from build123d import *

# Parameters (mm, degrees)
F1_DEPTH    = 200
F2_R        = 15
F4_DEPTH    = 15
F5_W        = 259.7017054144
F5_H        = 160
F6_DEPTH    = 50
F7_T1_DEPTH = 160
F8_R        = 15
F9_DEPTH    = 300


# Not quite as in the source:
# - a fillet or chamfer that OpenCascade refuses, or shapes differently, is made with other operations: its cross-section is extruded or revolved along the edge and cut away or added


with BuildPart() as f1:
    # F0 (on Front) → F1 (new body)
    with BuildSketch(Plane.XZ):
        with BuildLine():
            add(Edge.make_bspline(
                [(20.2008041868, 100), (146.0822657859, 99.5052919304), (265.431836351, 89.8162356005), (400, 75.4941478372)],
                knots=[0.5253173238, 0.5253173238, 0.5253173238, 0.5253173238, 1, 1, 1, 1], degree=3))
            Line((20.2008041868, 100), (0, 100))
            add(Edge.make_bspline(
                [(-400, 75.4941478372), (-275.3232982272, 88.4775108691), (-133.3944766528, 99.4743507493), (0, 100)],
                knots=[0, 0, 0, 0, 0.5, 0.5, 0.5, 0.5], degree=3))
            Line((-400, 75.4941478372), (-400, 44.4300249219))
            add(Edge.make_bspline(
                [(-41.6261814535, 0), (-214.6242707968, 0), (-393.6260249555, 49.33328574), (-400, 44.4300249219)],
                knots=[0, 0, 0, 0, 0.9473133281, 0.9473133281, 0.9473133281, 0.9473133281], degree=3))
            Line((-41.6261814535, 0), (209.8438292742, -64.8676306009))
            Line((209.8438292742, -64.8676306009), (266.6716873646, 0))
            add(Edge.make_bspline(
                [(400, 75.4941478372), (313.5865926743, 36.6108752787), (291.246175766, 29.9087464809), (266.6716873646, 0)],
                knots=[0, 0, 0, 0, 153.2181624608, 153.2181624608, 153.2181624608, 153.2181624608], degree=3))
        make_face()
    extrude(amount=F1_DEPTH)

    # F2
    f2_edges = [f1.edges().sort_by_distance(p)[0] for p in [
        (-200.289149, -200, 92.61289),
        (210.407204, -200, 92.68637),
        (-200.289149, 0, 92.61289),
        (10.100402, -200, 100),
        (10.100402, 0, 100),
        (210.407204, 0, 92.68637),
    ]]
    fillet(f2_edges, radius=F2_R)

    # F3 (on face) → F4 (cut, symmetric)
    with BuildSketch(Plane(origin=(150.8768626718, 0, -132.1770020211), x_dir=(0, 1, 0), z_dir=(0.7521818814, 0, -0.6589555503))):
        with BuildLine():
            Line((-180, 226.1682897806), (-180, 89.4854995586))
            Line((-180, 89.4854995586), (-20, 89.4854995586))
            Line((-20, 89.4854995586), (-20, 226.1682897806))
            add(Edge.make_bspline(
                [(-180, 226.1682897806), (-153.3333333333, 247.7404251695), (-100, 290.8846959472), (-46.6666666667, 247.7404251695), (-20, 226.1682897806)],
                knots=[0, 0, 0, 0, 0.5, 1, 1, 1, 1], degree=3))
        make_face()
    extrude(amount=F4_DEPTH, both=True, mode=Mode.SUBTRACT)

    # F5 (on face) → F6 (cut)
    with BuildSketch(Plane(origin=(-2.5970065182, 0, -10.0677217734), x_dir=(0.9683032706, 0, -0.2497774533), z_dir=(-0.2497774533, 0, -0.9683032706))):
        with Locations((89.5440850641, 100)):
            Rectangle(F5_W, F5_H)
    extrude(amount=-F6_DEPTH, mode=Mode.SUBTRACT)

    # F7: fillet of radius 15 on 1 edges, made by hand

    # F7_s2 → F7_t1 (cut)
    with BuildSketch(Plane.XZ.offset(20)):
        with BuildLine():
            ThreePointArc((236.54494855, -11.6256507443), (230.0859706945, -15.9445365763), (222.3327019401, -16.452467072))
            Line((222.3327019401, -16.452467072), (218.1662168076, -32.6045301468))
            Line((218.1662168076, -32.6045301468), (236.54494855, -11.6256507443))
        make_face()
    extrude(amount=F7_T1_DEPTH, mode=Mode.SUBTRACT)

    # F8 (on face) → F9 (cut)
    with BuildSketch(Plane.XZ.offset(200)):
        with Locations((198.1902569532, -39.8889631033)):
            Circle(F8_R)
    extrude(amount=-F9_DEPTH, mode=Mode.SUBTRACT)


solid = f1.part
Geometry check sheet. Reference: the model listing, model coordinates, mm. A direction names the side the tool comes from. Give positions to 0.01 mm unless a question says otherwise; leave off trailing zeros. Write each loop counter-clockwise with the first axis right and the second up, starting at its lowest first coordinate (ties: lowest second). Pieces come first, ordered by that corner, then holes. Notation, with made-up numbers: (49, -13) - (79, -13) arc R26 ccw to (79, 11) - close; hole circle Ø2 at (36, 55). An arc over 180 degrees is marked (long way). Put each result on its own line as item: value.
1. Thickness scan on line 1 (Y direction, x = 63, z = 2.5); line 2 (X direction, y = -68, z = 55.5); line 3 (X direction, y = -83, z = 59). Record the ranges inside material, lowest first.
Ans:
line 1: y = -200 to -180, -20 to 0
line 2: x = -400 to 295.35, 331.73 to 355.12
line 3: x = -400 to 298.42, 337.23 to 363
2. Set-up check for faces 1 (the flat face through (329.2, -100.83, 48.61)), 2 (the flat face through (-8, -200, 28)), 3 (the flat face through (-35.47, -98.88, 23.87)): record each of +Z, -Z, +X, -X, +Y, -Y from which the full face is reachable in a straight line by a thin tool's end or side.
Ans:
face 1: none
face 2: +Z, -Z, +X, -X, -Y
face 3: -Z
3. Sectioned sample at A-A, the plane x = 13. Enter the section's corners in (y, z), plus the area to 3 significant figures.
Ans:
outline: (-200, -14.09) - (-180, -14.09) - (-180, 37.55) - (-20, 37.55) - (-20, -14.09) - (0, -14.09) - (0, 85) arc R15 ccw to (-15, 100) - (-185, 100) arc R15 ccw to (-200, 85) - close
area: 14,500 mm²
4. Draft check along X on faces 4 (the flat face through (237.86, -189.86, -32.89)), 5 (the cylindrical face through (183.205, -190.14, -39.229)), 6 (the flat face through (-400, -99, 60)), 7 (the flat face through (274.047, -101.12, 31.182)). Enter one of: +X half, -X half, draft (parallel to the pull), parting line (faces both ways), or undercut.
Ans:
face 4: +X half
face 5: undercut
face 6: -X half
face 7: undercut
5. Go/stop test with flat-tipped pins: pin 1 (8 mm diameter, centred on y = -140.5, z = 15.5, fed in from +X); pin 2 (10 mm diameter, centred on y = -173, z = 55.5, fed in from +X); pin 3 (4 mm diameter, centred on y = -61, z = -3, fed in from +X). Record where each tip stops, or that it passes through.
Ans:
pin 1: stops at x = 263.81
pin 2: stops at x = 366.38
pin 3: stops at x = 245.85
